Autodesk Inventor part; units mm, degrees
ref_plane "YZ Plane" through (0, 0, 0) normal (1, 0, 0) x (0, 1, 0)
ref_plane "XZ Plane" through (0, 0, 0) normal (0, 1, 0) x (-1, 0, 0)
ref_plane "XY Plane" through (0, 0, 0) normal (0, 0, 1) x (1, 0, 0)
sketch "Sketch1" plane through (0, 0, 0) normal (0, 0, 1) x (1, 0, 0)
  line L0 (-100, 135) -> (140, 135)
  line L1 (140, 135) -> (140, -117.5)
  line L2 (140, -117.5) -> (-100, -117.5)
  line L3 (-100, -117.5) -> (-100, 135)
  point P0 (0, 0)
  dimension "d0" = 240
  dimension "d1" = 140
  dimension "d2" = 252.5
  dimension "d3" = 135
extrude "baseExtrusion" add sketch "Sketch1" along normal blind 10.2
sketch "Sketch2" plane through (0, 0, 10.2) normal (0, 0, 1) x (1, 0, 0)
  circle A0 centre (0, -52.5) radius 22.5
  line L0 (-100, -117.5) -> (140, -117.5)
  point P0 (0, 0)
  dimension "d6" = 45
  dimension "d7" = 65
extrude "objectiveExtrusion" cut sketch "Sketch2" against normal through all
sketch "Sketch3" plane through (0, 0, 10.2) normal (0, 0, 1) x (1, 0, 0)
  circle A0 centre (0, -52.5) radius 22.5
  point P0 (0, 0)
  point P1 (-30, -22.5)
  point P2 (30, -22.5)
  point P3 (-30, -82.5)
  point P4 (30, -82.5)
  dimension "d10" = 60
  dimension "d11" = 60
  dimension "d12" = 30
  dimension "d41" = 30
hole "60mmCageRodThread" at (-30, -22.5, 10.2) at (30, -22.5, 10.2) at (-30, -82.5, 10.2) at (30, -82.5, 10.2) direction (0, 0, -1) diameter 2.156 end through all
sketch "Sketch4" plane through (0, 0, 10.2) normal (0, 0, 1) x (1, 0, 0)
  circle A0 centre (0, -52.5) radius 22.5
  line L0 (-100, 135) -> (-100, -117.5)
  point P0 (0, 0)
  point P1 (-87.5, 117.5)
  point P2 (112.5, 117.5)
  point P3 (-87.5, 17.5)
  point P4 (112.5, 17.5)
  point P5 (12.5, 117.5)
  point P6 (-37.5, 117.5)
  point P7 (62.5, 117.5)
  point P8 (-87.5, -7.5)
  point P9 (112.5, -7.5)
  point P10 (-87.5, 67.5)
  dimension "d20" = 200
  dimension "d21" = 100
  dimension "d23" = 70
  dimension "d74" = 100
  dimension "d75" = 25
  dimension "d76" = 50
  dimension "d77" = 50
  dimension "d78" = 12.5
  dimension "d79" = 50
hole "m6BreadoardMountingHoles" at (-87.5, 117.5, 10.2) at (112.5, 117.5, 10.2) at (-87.5, 17.5, 10.2) at (112.5, 17.5, 10.2) at (12.5, 117.5, 10.2) at (-87.5, -7.5, 10.2) at (112.5, -7.5, 10.2) at (62.5, 117.5, 10.2) at (-37.5, 117.5, 10.2) at (-87.5, 67.5, 10.2) direction (0, 0, -1) diameter 6.6 end through all counterbore diameter 18 counterbore depth 4.8
sketch "Sketch5" plane through (0, 0, 0) normal (0, 0, -1) x (-1, 0, 0)
  circle A0 centre (0, -52.5) radius 22.5
  point P0 (0, 0)
  point P1 (-8.4, 57.5)
  point P2 (-107.3, 67.7)
  dimension "d31" = 110
  dimension "d40" = 8.4
  dimension "d72" = 98.9
  dimension "d73" = 10.2
hole "m4MirrorTLMountingHoles" at (8.4, 57.5, 0) at (107.3, 67.7, 0) direction (0, 0, 1) diameter 4.5 end through all counterbore diameter 13 counterbore depth 3.4
sketch "Sketch6" plane through (0, 0, 10.2) normal (0, 0, 1) x (1, 0, 0)
  circle A0 centre (-30, -22.5) radius 1.078
  point P0 (0, 0)
  point P1 (-60, -5)
  point P2 (60, -5)
  point P3 (-60, -52.5)
  point P4 (60, -52.5)
  point P5 (0, -107.5)
  dimension "d42" = 120
  dimension "d43" = 60
  dimension "d44" = 47.5
  dimension "d45" = 55
  dimension "d46" = 30
hole "m6objectiveHolderMountingHoles" at (-60, -5, 10.2) at (60, -5, 10.2) at (-60, -52.5, 10.2) at (60, -52.5, 10.2) at (0, -107.5, 10.2) direction (0, 0, -1) diameter 4.917 end through all
sketch "Sketch7" plane through (0, 0, 0) normal (0, 0, -1) x (-1, 0, 0)
  circle A0 centre (0, -52.5) radius 22.5
  point P0 (0, 0)
  point P1 (-24.25, 15.5)
  point P2 (24.25, 15.5)
  dimension "d54" = 48.5
  dimension "d55" = 24.25
  dimension "d56" = 68
hole "filterwheelMountingHoles" at (24.25, 15.5, 0) at (-24.25, 15.5, 0) direction (0, 0, 1) diameter 6.6 depth 17.1 tip angle 118 counterbore diameter 10 counterbore depth 4.8
properties part number "detectionObjHolder"
Check sheet for the modelled part. Datum: model origin and axes. Units: mm. A direction names the side the tool comes from. Round coordinates to 2 decimals unless told otherwise and drop trailing zeros. Write item = value, one per line. Start each with the question number.
1. Gauge pin test, flat ends, axial feed: pin 1 (9 mm diameter, centred on x = -86, y = 20, fed in from +Z); pin 2 (23.5 mm diameter, centred on x = -87.5, y = 67.5, fed in from +Z). Record the tip position at first contact, or that the pin passes through.
2. Tool access check on faces 1 (the cylindrical face through (107.014, 61.206, 1.724)), 2 (the flat face through (-88, 14, 5.4)), 3 (the cylindrical face through (112.4, 20.8, 2.7)). Record the directions out of +Z, -Z, +X, -X, +Y, -Y that give a thin tool (end or side, any length) a straight path to the whole face; none if there is none.
3. Scan lines: line 1 (X direction, y = 117.5, z = 1.2); line 2 (X direction, y = -82.5, z = 2.5); line 3 (Y direction, x = -30, z = 4). Record each from-to range of solid material in increasing order. Write a range as [from, to].
4. Release check for a two-part mould opening along Y. For faces 4 (the cylindrical face through (-78.714, 19.451, 7.766)), 5 (the flat face through (18, 11, 0)) record: pulls with the +Y half, pulls with the -Y half, needs draft (parallel to the pull), parting line crosses it, or undercut.
5. Section check A-A, the plane z = 1.75. State how many separate pieces and enclosed holes the cut face has, then the cut area to 3 significant figures.
Results found:
q1.pin_1 = 5.4
q1.pin_2 = 10.2
q2.face_1 = -Z
q2.face_2 = +Z
q2.face_3 = +Z, -Z
q3.line_1 = [-100, -90.8], [-84.2, -40.8], [-34.2, 9.2], [15.8, 59.2], [65.8, 109.2], [115.8, 140]
q3.line_2 = [-100, -31.08], [-28.92, 28.92], [31.08, 140]
q3.line_3 = [-117.5, -83.58], [-81.42, -23.58], [-21.42, 135]
q4.face_4 = undercut
q4.face_5 = needs draft
q5.separate_pieces = 1
q5.enclosed_holes = 24
q5.area = 58,100 mm^2
